Verification items for the finished model (mm, model axes). Face numbers are marked on the shaded views. A direction names the side the tool comes from. Give positions to 0.01 mm unless a question says otherwise; leave off trailing zeros. Order: outer loops, then holes, each group sorted by start corner. A loop starts at its lowest first (then second) coordinate and runs counter-clockwise, first axis right, second up.
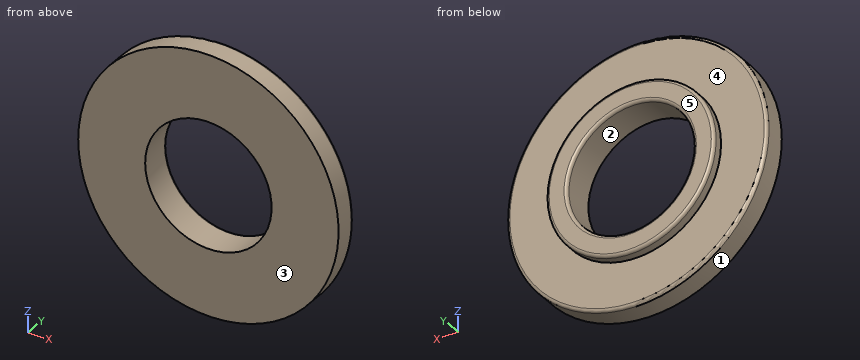
Autodesk Inventor part; units mm, degrees
ref_plane "YZ Plane" through (0, 0, 0) normal (1, 0, 0) x (0, 1, 0)
ref_plane "XZ Plane" through (0, 0, 0) normal (0, 1, 0) x (-1, 0, 0)
ref_plane "XY Plane" through (0, 0, 0) normal (0, 0, 1) x (1, 0, 0)
sketch "Sketch1" plane through (0, 0, 0) normal (0, 1, 0) x (-1, 0, 0)
  circle A0 centre (0, 0) radius 8.75
  circle A1 centre (0, 0) radius 5.65
  circle A2 centre (0, 0) radius 4.25
  dimension "d0" = 17.5
  dimension "d1" = 11.3
  dimension "d2" = 8.5
extrude "Extrusion1" add sketch "Sketch1" along normal blind 2.2 contours A1
extrude "Extrusion2" add sketch "Sketch1" along normal blind 1.5 contours A0
fillet "Fillet1" radius 0.2 3 edges at (4.25, 2.2, 0) (5.65, 2.2, 0) (8.75, 1.5, 0)
properties part number "ZKE-Term-Solid-Shim" material "ABS Plastic"
(1) Scan lines: line 1 (Z direction, x = 0, y = 0.55); line 2 (X direction, y = 2.1, z = 2.5); line 3 (Y direction, x = 7.25, z = 1). Record each from-to range of solid material in increasing order.
Solved:
line 1: z = -8.75 to -4.25, 4.25 to 8.75
line 2: x = -5.04 to -3.47, 3.47 to 5.04
line 3: y = 0 to 1.5
(2) Section check B-B, the plane z = 0. Enter the section's corners in (x, y), then the cut area to 3 significant figures.
Solved:
outline: (-8.75, 0) - (-4.25, 0) - (-4.25, 2) arc R0.2 ccw to (-4.45, 2.2) - (-5.45, 2.2) arc R0.2 ccw to (-5.65, 2) - (-5.65, 1.5) - (-8.55, 1.5) arc R0.2 ccw to (-8.75, 1.3) - close; (4.25, 0) - (8.75, 0) - (8.75, 1.3) arc R0.2 ccw to (8.55, 1.5) - (5.65, 1.5) - (5.65, 2) arc R0.2 ccw to (5.45, 2.2) - (4.45, 2.2) arc R0.2 ccw to (4.25, 2) - close
area: 15.4 mm2
(3) Go/stop test with a flat-tipped pin: pin 1 (8 mm diameter, centred on x = 5.5, z = -1.5, fed in from -Y). Record where the tip stops, or that it passes through.
Solved:
pin 1: stops at y = 0
(4) Set-up check for the marked faces 4 and 5: record each of +Z, -Z, +X, -X, +Y, -Y from which the full face is reachable in a straight line by a thin tool's end or side.
Solved:
face 4: +Y
face 5: +Z, -Z, +X, -X, +Y
(5) Section check C-C, the plane y = 0.7. Enter the section's corners in (x, z).
Solved:
outline: circle Ø17.5 at (0, 0); hole circle Ø8.5 at (0, 0)
(6) Section check A-A, the plane x = 0. Enter the section's corners in (y, z).
Solved:
outline: (0, -8.75) - (1.3, -8.75) arc R0.2 ccw to (1.5, -8.55) - (1.5, -5.65) - (2, -5.65) arc R0.2 ccw to (2.2, -5.45) - (2.2, -4.45) arc R0.2 ccw to (2, -4.25) - (0, -4.25) - close; (0, 4.25) - (2, 4.25) arc R0.2 ccw to (2.2, 4.45) - (2.2, 5.45) arc R0.2 ccw to (2, 5.65) - (1.5, 5.65) - (1.5, 8.55) arc R0.2 ccw to (1.3, 8.75) - (0, 8.75) - close
(7) Release check for a two-part mould opening along X. For the marked faces 1, 2 and 3 record: pulls with the +X half, pulls with the -X half, needs draft (parallel to the pull), parting line crosses it, or undercut.
Solved:
face 1: parting line crosses it
face 2: undercut
face 3: needs draft
